The listing builds one solid part. Answer for the finished solid, in the listing's coordinates (mm). A direction names the side the tool comes from. Give positions to 0.01 mm unless a question says otherwise; leave off trailing zeros. Write each loop counter-clockwise with the first axis right and the second up, starting at its lowest first coordinate (ties: lowest second). Pieces come first, ordered by that corner, then holes. Notation, with made-up numbers: (-1, 89.5) - (53, 89.5) arc R15 cw to (53, 106.5) - close; hole circle Ø5 at (-17, 9.25). An arc over 180 degrees is marked (long way). Use a Markdown table: item, result. Add a question column.
from build123d import *

# Parameters (mm, degrees)
F0_W     = 18
F0_H     = 120
F1_DEPTH = 115
F2_R     = 10
F3_W     = 200
F3_H     = 113
F4_DEPTH = 500.001
F5_W     = 18.0844597816
F5_H     = 229.7550716996
F5_W_2   = 18.6774961948
F5_H_2   = 230
F6_DEPTH = 5


with BuildPart() as f1:
    # F0 (on Front) → F1 (new body, symmetric)
    with BuildSketch(Plane.XZ):
        Polygon((250, 9), (-250, 9), (-250, -9), (-232, -9), (232, -9), (250, -9), align=None)
        with Locations((-241, -69)):
            Rectangle(F0_W, F0_H)
        with Locations((241, -69)):
            Rectangle(F0_W, F0_H)
    extrude(amount=F1_DEPTH, both=True)

    # F2
    f2_edges = [f1.edges().sort_by_distance(p)[0] for p in [
        (-250, 0, 9),
        (250, 0, 9),
    ]]
    fillet(f2_edges, radius=F2_R)

    # F3 (on face) → F4 (cut, through all)
    with BuildSketch(Plane.YZ.offset(250)):
        with Locations((0, -72.5)):
            Rectangle(F3_W, F3_H)
    extrude(amount=-F4_DEPTH, mode=Mode.SUBTRACT)

    # F5 (on face) → F6 (join)
    with BuildSketch(Plane(origin=(0, 0, -9), x_dir=(1, 0, 0), z_dir=(0, 0, -1))):
        with Locations((-241.0422298908, -0.1224641502)):
            Rectangle(F5_W, F5_H)
        with Locations((241.3387480974, 0)):
            Rectangle(F5_W_2, F5_H_2)
    extrude(amount=F6_DEPTH)


solid = f1.part
1. For a pull along Y with two mould halves and no side action, classify faces 4 (the flat face through (-0.8, -115, -8.6)), 5 (the flat face through (-241, -100, -73)), 6 (the flat face through (241, 107, -129)) as released by +Y, released by -Y, zero draft, split by the parting line, or undercut.
2. Which of the six approach directions +Z, -Z, +X, -X, +Y, -Y give full straight-line access (tool end or side, diameter ignored) to faces 1 (the flat face through (-241, 100, -73)), 2 (the flat face through (-232, 8, -12)), 3 (the flat face through (250, 102, -76))?
3. The part is cut by section C-C (x = 175). Give the vertices of the cut face in (y, z), and give its area (3 significant figures).
4. Given P1, Ø0.7, axis at x = 250, y = -7.5, coming from the -Z side; P2, Ø9, axis at y = 28.5, z = -3.5, coming from the +X side; P3, Ø4, axis at x = 7.5, y = 38, coming from the -Z side, each flat-ended and moving along its own axis, determine where each tip first touches the part or whether it passes through.
5. The part is cut by section A-A (z = -22). Give the vertices of the cut face in (x, y).
6. The part is cut by section B-B (y = 94). Give the vertices of the cut face in (x, z).
7. Consider L1, parallel to X at y = -16.5, z = -15.5; L2, parallel to X at y = -7.5, z = -11; L3, parallel to Z at x = -63, y = -3.5. Determine where each line is inside the solid, lowest interval first. Write a range as [from, to].
Check values:
| question | item | result |
|---|---|---|
| 1 | face 4 | released by -Y |
| 1 | face 5 | undercut |
| 1 | face 6 | zero draft |
| 2 | face 1 | -Z, +X, -X |
| 2 | face 2 | -Z, +Y, -Y |
| 2 | face 3 | -Z, +X, +Y, -Y |
| 3 | outline | (-115, -9) - (115, -9) - (115, 9) - (-115, 9) - close |
| 3 | area | 4,140 mm2 |
| 4 | P1 | stops at z = -16 |
| 4 | P2 | stops at x = 250 |
| 4 | P3 | stops at z = -9 |
| 5 | outline | (-250, -115) - (-232, -115) - (-232, -100) - (-250, -100) - close; (-250, 100) - (-232, 100) - (-232, 115) - (-250, 115) - close; (232, -115) - (250, -115) - (250, -100) - (232, -100) - close; (232, 100) - (250, 100) - (250, 115) - (232, 115) - close |
| 6 | outline | (-250.08, -14) - (-250, -14) - (-250, -16) - (-232, -16) - (-232, -9) - (232, -9) - (232, -16) - (250, -16) - (250, -14) - (250.68, -14) - (250.68, -9) - (250, -9) - (250, -1) arc R10 ccw to (240, 9) - (-240, 9) arc R10 ccw to (-250, -1) - (-250, -9) - (-250.08, -9) - close |
| 7 | L1 | x = [-250, -232], [232, 250] |
| 7 | L2 | x = [-250.08, -232], [232, 250.68] |
| 7 | L3 | z = [-9, 9] |
